Check sheet for the modelled part. Datum: model origin and axes. Units: mm. A direction names the side the tool comes from. Coordinates: 2 decimals unless noted, no trailing zeros. Loops run counter-clockwise (first coordinate to the right, second up) from the corner with the lowest first, then second, coordinate; pieces in that order, holes last. Notation, with made-up numbers: (-30.75, 60) - (-0.75, 60) arc R33 ccw to (-0.75, 96) - close; hole circle Ø6 at (23.25, 50.5). An arc over 180 degrees is marked (long way). Use a Markdown table: item, result. Add a question column.
1) Go/stop test with flat-tipped pins: P1, Ø2.5, axis at x = -24, z = -4, coming from the -Y side; P2, Ø0.9, axis at y = 18, z = -2, coming from the -X side; P3, Ø2, axis at x = -12, z = -26.5, coming from the +Y side. Record where each tip stops, or that it passes through.
2) Sectioned sample at C-C, the plane y = 17.5. Enter the section's corners in (x, z).
3) Sectioned sample at D-D, the plane x = -14. Enter the section's corners in (y, z).
4) Sectioned sample at B-B, the plane x = 2.5. Enter the section's corners in (y, z).
5) Tool access check on faces 1 (the flat face through (-22.854, 18, -11)), 2 (the flat face through (13, 16, -11)), 3 (the cylindrical face through (-14.695, 12.605, -22.276)). Record the directions out of +Z, -Z, +X, -X, +Y, -Y that give a thin tool (end or side, any length) a straight path to the whole face; none if there is none.
6) Draft check along X on faces 4 (the flat face through (-13, 5, -26)), 5 (the cylindrical face through (2.7, 12.6, -22.17)), 6 (the flat face through (14.146, 19.5, -11.2)), 7 (the flat face through (-6, 10, -31.509)). Enter one of: pulls with the +X half, pulls with the -X half, needs draft (parallel to the pull), parting line crosses it, or undercut.
7) Sectioned sample at A-A, the plane z = -20. Enter the section's corners in (x, y), then the cut area to 3 significant figures.
8) Thickness scan on line 1 (Z direction, x = -15, y = 16.5); line 2 (X direction, y = 10, z = -28.5); line 3 (Y direction, x = 1, z = -24). Record the ranges inside material, lowest first.
from build123d import *

# Parameters (mm, degrees)
SKETCH1_W           = 40
SKETCH1_H           = 40
BOSS_EXTRUDE1_DEPTH = 20
SKETCH2_R           = 3.5
CUT_EXTRUDE1_DEPTH  = 15
SKETCH3_W           = 40
SKETCH3_H           = 3
CUT_EXTRUDE2_DEPTH  = 3


with BuildPart() as part:
    # Sketch1 → Boss-Extrude1 (new body)
    with BuildSketch(Plane(origin=(0, 0, 0), x_dir=(1, 0, 0), z_dir=(0, 1, 0))):
        with Locations((-5.853997969, 11.508758813)):
            Rectangle(SKETCH1_W, SKETCH1_H)
    extrude(amount=BOSS_EXTRUDE1_DEPTH)

    # Sketch2 → Cut-Extrude1 (cut)
    with BuildSketch(Plane(origin=(0, 20, 0), x_dir=(1, 0, 0), z_dir=(0, 1, 0))):
        with Locations(Location((-13.353997969, 25.508758813, 0), (0, 0, 270))):
            Circle(SKETCH2_R)
        with Locations(Location((1.646002031, 25.508758813, 0), (0, 0, 270))):
            Circle(SKETCH2_R)
    extrude(amount=-CUT_EXTRUDE1_DEPTH, mode=Mode.SUBTRACT)

    # Sketch3 → Cut-Extrude2 (cut)
    with BuildSketch(Plane(origin=(14.146002031, 0, 0), x_dir=(0, 0, -1), z_dir=(1, 0, 0))):
        with Locations((11.508758813, 17.5)):
            Rectangle(SKETCH3_W, SKETCH3_H)
    cut_extrude2 = extrude(amount=-CUT_EXTRUDE2_DEPTH, mode=Mode.SUBTRACT)

    # Mirror1: Cut-Extrude2 across plane
    add(cut_extrude2.mirror(Plane(origin=(-5.853997969, 0, 0), x_dir=(0, 0, 1), z_dir=(1, 0, 0))), mode=Mode.SUBTRACT)


solid = part.part
Solved:
| question | item | result |
|---|---|---|
| 1 | P1 | stops at y = 0 |
| 1 | P2 | stops at x = -22.85 |
| 1 | P3 | stops at y = 5 |
| 2 | outline | (-22.85, -31.51) - (11.15, -31.51) - (11.15, 8.49) - (-22.85, 8.49) - close; hole circle Ø7 at (-13.35, -25.51); hole circle Ø7 at (1.65, -25.51) |
| 3 | outline | (0, -31.51) - (20, -31.51) - (20, -28.95) - (5, -28.95) - (5, -22.07) - (20, -22.07) - (20, 8.49) - (0, 8.49) - close |
| 4 | outline | (0, -31.51) - (20, -31.51) - (20, -28.9) - (5, -28.9) - (5, -22.11) - (20, -22.11) - (20, 8.49) - (0, 8.49) - close |
| 5 | face 1 | +Z, -Z, -X |
| 5 | face 2 | +Z, -Z, +X |
| 5 | face 3 | +Y |
| 6 | face 4 | undercut |
| 6 | face 5 | undercut |
| 6 | face 6 | pulls with the +X half |
| 6 | face 7 | needs draft |
| 7 | outline | (-25.85, 0) - (14.15, 0) - (14.15, 16) - (11.15, 16) - (11.15, 19) - (14.15, 19) - (14.15, 20) - (-25.85, 20) - (-25.85, 19) - (-22.85, 19) - (-22.85, 16) - (-25.85, 16) - close |
| 7 | area | 782 mm2 |
| 8 | line 1 | z = -31.51 to -28.6, -22.42 to 8.49 |
| 8 | line 2 | x = -25.85 to -15.17, -11.54 to -0.17, 3.46 to 14.15 |
| 8 | line 3 | y = 0 to 5 |
